```python
from build123d import *

# Parameters (mm, degrees)
SKETCH1_R           = 22.5
BOSS_EXTRUDE1_DEPTH = 7
CUT_EXTRUDE1_DEPTH  = 8
CIRPATTERN1_COUNT   = 24
SKETCH3_R           = 5
BOSS_EXTRUDE2_DEPTH = 7
SKETCH4_R           = 2
CUT_EXTRUDE2_DEPTH  = 15
SKETCH5_R           = 2
CUT_EXTRUDE3_DEPTH  = 23.360679775


with BuildPart() as part:
    # Sketch1 → Boss-Extrude1 (new body)
    with BuildSketch(Plane(origin=(0, 0, 0), x_dir=(1, 0, 0), z_dir=(0, 1, 0))):
        Circle(SKETCH1_R)
    extrude(amount=BOSS_EXTRUDE1_DEPTH)

    # Sketch2 → Cut-Extrude1 (cut, through all)
    with BuildSketch(Plane(origin=(0, 7, 0), x_dir=(1, 0, 0), z_dir=(0, 1, 0))):
        with BuildLine():
            ThreePointArc((2.5, 22.360679775), (1.560955546, 20.431571445), (1, 18.360679775))
            ThreePointArc((1, 18.360679775), (0, 18.387891717), (-1, 18.360679775))
            ThreePointArc((-1, 18.360679775), (-1.560955546, 20.431571445), (-2.5, 22.360679775))
            ThreePointArc((-2.5, 22.360679775), (0, 22.5), (2.5, 22.360679775))
        make_face()
    cut_extrude1 = extrude(amount=-CUT_EXTRUDE1_DEPTH, mode=Mode.SUBTRACT)

    # CirPattern1: Cut-Extrude1 ×24 about axis
    cirpattern1_axis = Axis((0, 0, 0), (0, 1, 0))
    for i in range(1, CIRPATTERN1_COUNT):
        add(cut_extrude1.rotate(cirpattern1_axis, i * 360 / CIRPATTERN1_COUNT), mode=Mode.SUBTRACT)

    # Sketch3 → Boss-Extrude2 (add)
    with BuildSketch(Plane(origin=(0, 7, 0), x_dir=(1, 0, 0), z_dir=(0, 1, 0))):
        Circle(SKETCH3_R)
    extrude(amount=BOSS_EXTRUDE2_DEPTH)

    # Sketch4 → Cut-Extrude2 (cut, through all)
    with BuildSketch(Plane(origin=(0, 14, 0), x_dir=(1, 0, 0), z_dir=(0, 1, 0))):
        Circle(SKETCH4_R)
    extrude(amount=-CUT_EXTRUDE2_DEPTH, mode=Mode.SUBTRACT)

    # Sketch5 → Cut-Extrude3 (cut, through all)
    with BuildSketch(Plane.XY):
        with Locations((0, 10.5)):
            Circle(SKETCH5_R)
    extrude(amount=-CUT_EXTRUDE3_DEPTH, mode=Mode.SUBTRACT)


solid = part.part
```
Input: part model. Units: mm. Frame: model coordinates. A direction names the side the tool comes from. Round coordinates to 2 decimals unless told otherwise and drop trailing zeros. Write each loop counter-clockwise with the first axis right and the second up, starting at its lowest first coordinate (ties: lowest second). Pieces come first, ordered by that corner, then holes. Notation, with made-up numbers: (21.5, -2.5) -> (68.5, -2.5) arc R11 cw to (68.5, 9.5) -> close; hole circle Ø4 at (10.5, 54.5). An arc over 180 degrees is marked (long way). Answer as CSV lines item,"result".
1. Contact query for flat-ended pins moving along their axis: P1, Ø8, axis at y = 3, z = -16.5, coming from the +X side; P2, Ø1, axis at y = 10.5, z = -3.5, coming from the -X side; P3, Ø8, axis at x = 11.5, y = 2, coming from the +Z side. Output: stop coordinate, or through.
Geometry says:
P1,"stops at x = 18.11"
P2,"stops at x = -4"
P3,"stops at z = 20.95"
2. Section C-C (z = -7.5). Return the cut outline in (x, y), plus the area to 3 significant figures.
Geometry says:
outline,"(-20.22, 0) -> (20.22, 0) -> (20.22, 7) -> (-20.22, 7) -> close"
area,"283 mm^2"
3. Mould query, pull axis Z, two halves, no side actions, for faces 5 (the cylindrical face through (-1.57, 3.55, 20.46)), 6 (the cylindrical face through (16.93, 3.55, 11.59)), 7 (the cylindrical face through (-6.78, 3.55, -19.31)). Classes: +Z half, -Z half, draft (parallel to the pull), parting line (faces both ways), or undercut.
Geometry says:
face 5,"+Z half"
face 6,"undercut"
face 7,"-Z half"
4. Ray query, L1, parallel to Z at x = 16, y = 2.25; L2, parallel to Z at x = 19.5, y = 6; L3, parallel to Y at x = 18, z = -0.5. Return the intervals inside material, ascending. Write a range as [from, to].
Geometry says:
L1,"z = [-13.54, -10.58], [-9.06, 9.06], [10.58, 13.54]"
L2,"z = [-8.99, -6.92], [-3.82, -1.26], [1.26, 3.82], [6.92, 8.99]"
L3,"y = [0, 7]"
5. Section A-A (x = 0). Return the cut outline in (y, z).
Geometry says:
outline,"(0, -18.39) -> (7, -18.39) -> (7, -5) -> (8.5, -5) -> (8.5, -2) -> (0, -2) -> close; (0, 2) -> (14, 2) -> (14, 5) -> (7, 5) -> (7, 18.39) -> (0, 18.39) -> close; (12.5, -5) -> (14, -5) -> (14, -2) -> (12.5, -2) -> close"
6. Section B-B (x = 7). Return the cut outline in (y, z), plus the area to 3 significant figures.
Geometry says:
outline,"(0, -19.61) -> (7, -19.61) -> (7, 19.61) -> (0, 19.61) -> close"
area,"275 mm^2"
7. Reachability of faces 1 (the cylindrical face through (19.31, 3.55, -6.78)), 2 (the cylindrical face through (-12.992, 3.549, -13.012)), 3 (the cylindrical face through (6.78, 3.55, 19.31)), 4 (the cylindrical face through (1.57, 3.55, -20.46)) from +Z, -Z, +X, -X, +Y, -Y: full face, straight path, thin tool, end or side. Return the list, or none.
Geometry says:
face 1,"+X, +Y, -Y"
face 2,"+Y, -Y"
face 3,"+Z, +Y, -Y"
face 4,"-Z, +Y, -Y"
